Geometry check sheet. Reference: the model listing, model coordinates, mm. Face numbers are marked on the shaded views. A direction names the side the tool comes from. Give positions to 0.01 mm unless a question says otherwise; leave off trailing zeros. Order: outer loops, then holes, each group sorted by start corner. A loop starts at its lowest first (then second) coordinate and runs counter-clockwise, first axis right, second up.
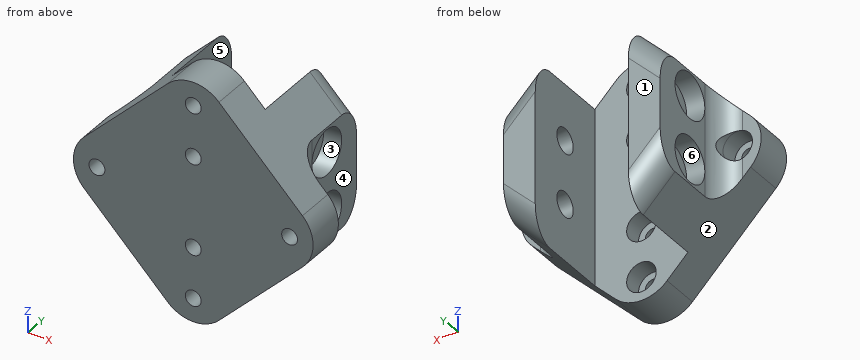
from build123d import *

# Parameters (mm, degrees)
SKETCH_1_R          = 1.75
EXTRUDE_1_DEPTH     = 8.5
EXTRUDE_2_DEPTH     = 20
SKETCH_3_R          = 2.75
CUT_EXTRUDE_1_DEPTH = 59.415752368
SKETCH_4_R          = 5
CUT_EXTRUDE_2_DEPTH = 4
SKETCH_5_R          = 3.25
CUT_EXTRUDE_3_DEPTH = 4
FILLET_2_R          = 5


with BuildPart() as part:
    # Эскиз1 → Бобышка-Вытянуть1 (new body)
    with BuildSketch(Plane(origin=(0, 0, 0), x_dir=(1, 0, 0), z_dir=(0, 1, 0))):
        with BuildLine():
            Line((5.656854249, -24.04163056), (24.04163056, -5.656854249))
            ThreePointArc((24.04163056, -5.656854249), (26.384776311, 0), (24.04163056, 5.656854249))
            Line((24.04163056, 5.656854249), (5.656854249, 24.04163056))
            ThreePointArc((5.656854249, 24.04163056), (0, 26.384776311), (-5.656854249, 24.04163056))
            Line((-5.656854249, 24.04163056), (-24.04163056, 5.656854249))
            ThreePointArc((-24.04163056, 5.656854249), (-26.384776311, 0), (-24.04163056, -5.656854249))
            Line((-24.04163056, -5.656854249), (-5.656854249, -24.04163056))
            ThreePointArc((-5.656854249, -24.04163056), (0, -26.384776311), (5.656854249, -24.04163056))
        make_face()
        with Locations(Location((21.213203436, 0, 0), (0, 0, 270))):
            Circle(SKETCH_1_R, mode=Mode.SUBTRACT)
        with Locations(Location((0, -10, 0), (0, 0, 270))):
            Circle(SKETCH_1_R, mode=Mode.SUBTRACT)
        with Locations(Location((0, -21.213203436, 0), (0, 0, 270))):
            Circle(SKETCH_1_R, mode=Mode.SUBTRACT)
        with Locations(Location((-21.213203436, 0, 0), (0, 0, 270))):
            Circle(SKETCH_1_R, mode=Mode.SUBTRACT)
        with Locations(Location((0, 10, 0), (0, 0, 270))):
            Circle(SKETCH_1_R, mode=Mode.SUBTRACT)
        with Locations(Location((0, 21.213203436, 0), (0, 0, 270))):
            Circle(SKETCH_1_R, mode=Mode.SUBTRACT)
    extrude(amount=EXTRUDE_1_DEPTH)

    # Эскиз2 → Бобышка-Вытянуть2 (add)
    with BuildSketch(Plane(origin=(0, 8.5, 0), x_dir=(1, 0, 0), z_dir=(0, 1, 0))):
        Polygon((-10.25, 19.44848481), (-10.25, -19.44848481), (-17.25, -12.44848481), (-17.25, 12.44848481), align=None)
        Polygon((17.25, 12.44848481), (10.25, 19.44848481), (10.25, -19.44848481), (17.25, -12.44848481), align=None)
    extrude(amount=EXTRUDE_2_DEPTH)

    # Эскиз3 → Вырез-Вытянуть1 (cut, through all)
    with BuildSketch(Plane(origin=(17.25, 0, 0), x_dir=(0, 0, -1), z_dir=(1, 0, 0))):
        with Locations((-7, 18.5)):
            Circle(SKETCH_3_R)
        with Locations((7, 18.5)):
            Circle(SKETCH_3_R)
    extrude(amount=-CUT_EXTRUDE_1_DEPTH, mode=Mode.SUBTRACT)

    # Эскиз4 → Вырез-Вытянуть2 (cut)
    with BuildSketch(Plane(origin=(17.25, 0, 0), x_dir=(0, 0, -1), z_dir=(1, 0, 0))):
        with Locations((-7, 18.5)):
            Circle(SKETCH_4_R)
        with Locations((7, 18.5)):
            Circle(SKETCH_4_R)
    cut_extrude_2 = extrude(amount=-CUT_EXTRUDE_2_DEPTH, mode=Mode.SUBTRACT)

    # Зеркальное отражение1: Вырез-Вытянуть2 across plane
    add(cut_extrude_2.mirror(Plane(origin=(0, 0, 0), x_dir=(0, 0, 1), z_dir=(1, 0, 0))), mode=Mode.SUBTRACT)

    # Эскиз5 → Вырез-Вытянуть3 (cut)
    with BuildSketch(Plane(origin=(0, 8.5, 0), x_dir=(1, 0, 0), z_dir=(0, 1, 0))):
        with Locations(Location((0, 21.213203436, 0), (0, 0, 270))):
            Circle(SKETCH_5_R)
        with Locations(Location((0, 10, 0), (0, 0, 270))):
            Circle(SKETCH_5_R)
        with Locations(Location((0, -10, 0), (0, 0, 270))):
            Circle(SKETCH_5_R)
        with Locations(Location((0, -21.213203436, 0), (0, 0, 270))):
            Circle(SKETCH_5_R)
        with Locations(Location((21.213203436, 0, 0), (0, 0, 270))):
            Circle(SKETCH_5_R)
        with Locations(Location((-21.213203436, 0, 0), (0, 0, 270))):
            Circle(SKETCH_5_R)
    extrude(amount=-CUT_EXTRUDE_3_DEPTH, mode=Mode.SUBTRACT)

    # Скругление2
    # the kernel refuses this fillet: 5 mm, written as the material it adds along each edge
    with BuildSketch(Plane(origin=(-17.25, 8.5, 24.94848481), x_dir=(-1, 0, 0), z_dir=(0, 0, -1))) as fillet_2_piece_1_section:
        with BuildLine():
            CenterArc((FILLET_2_R, FILLET_2_R), FILLET_2_R, 180, 90)
            Line((0, FILLET_2_R), (0, 0))
            Line((0, 0), (FILLET_2_R, 0))
        make_face()
    fillet_2_piece_1 = extrude(amount=49.89696962, mode=Mode.PRIVATE)
    fillet_2_piece_1 = split(fillet_2_piece_1, bisect_by=Plane(origin=(-29.470144139, 8.621513924, 0.22834067), z_dir=(0.7071067811865474, 0, -0.7071067811865477)), keep=Keep.TOP, mode=Mode.PRIVATE)
    fillet_2_piece_1 = split(fillet_2_piece_1, bisect_by=Plane(origin=(-21.171154266, 8.621513924, -8.527330544), z_dir=(0.7071067811865477, 0, 0.7071067811865474)), keep=Keep.TOP, mode=Mode.PRIVATE)
    fillet_2_piece_1 = fillet_2_piece_1 - Plane(origin=(-21.213203436, 8.621513924, 0), x_dir=(0, 0, 1), z_dir=(0, 1, 0)) * Cylinder(3.25, 120, mode=Mode.PRIVATE)
    add(fillet_2_piece_1)
    with BuildSketch(Plane(origin=(17.25, 8.5, 24.94848481), x_dir=(0, 1, 0), z_dir=(0, 0, -1))) as fillet_2_piece_2_section:
        with BuildLine():
            CenterArc((FILLET_2_R, FILLET_2_R), FILLET_2_R, 180, 90)
            Line((0, FILLET_2_R), (0, 0))
            Line((0, 0), (FILLET_2_R, 0))
        make_face()
    fillet_2_piece_2 = extrude(amount=49.89696962, mode=Mode.PRIVATE)
    fillet_2_piece_2 = split(fillet_2_piece_2, bisect_by=Plane(origin=(27.68449432, 12.192813605, 2.013990489), z_dir=(-0.7071067811865477, 0, -0.7071067811865474)), keep=Keep.TOP, mode=Mode.PRIVATE)
    fillet_2_piece_2 = split(fillet_2_piece_2, bisect_by=Plane(origin=(19.385504447, 12.192813605, -10.312980363), z_dir=(-0.7071067811865472, 0, 0.7071067811865478)), keep=Keep.TOP, mode=Mode.PRIVATE)
    fillet_2_piece_2 = fillet_2_piece_2 - Plane(origin=(21.213203436, 12.192813605, 0), x_dir=(0, 0, 1), z_dir=(0, 1, 0)) * Cylinder(3.25, 120, mode=Mode.PRIVATE)
    add(fillet_2_piece_2)
    # the kernel refuses this fillet: 5 mm, written as the material it takes off along each edge
    with BuildSketch(Plane(origin=(-26.088834765, 28.5, -3.609650045), x_dir=(0, -1, 0), z_dir=(0.7071067811865472, 0, -0.7071067811865478)), Plane(origin=(1.411165235, 28.5, 28.287319575), x_dir=(-0.7071067811865474, 0, -0.7071067811865477), z_dir=(0.7071067811865477, 0, -0.7071067811865474))) as fillet_2_2_piece_1:
        with BuildLine():
            CenterArc((FILLET_2_R, -FILLET_2_R), FILLET_2_R, 90, 90)
            Line((0, -FILLET_2_R), (0, 0))
            Line((0, 0), (FILLET_2_R, 0))
        make_face()
    extrude(amount=34.899494937, mode=Mode.SUBTRACT)
    with BuildSketch(Plane(origin=(-1.411165235, 28.5, 28.287319575), x_dir=(0.7071067811865474, 0, -0.7071067811865477), z_dir=(-0.7071067811865477, 0, -0.7071067811865474)), Plane(origin=(26.088834765, 28.5, -3.609650045), x_dir=(0, -1, 0), z_dir=(-0.7071067811865472, 0, -0.7071067811865478))) as fillet_2_2_piece_2:
        with BuildLine():
            CenterArc((FILLET_2_R, FILLET_2_R), FILLET_2_R, 180, 90)
            Line((0, FILLET_2_R), (0, 0))
            Line((0, 0), (FILLET_2_R, 0))
        make_face()
    extrude(amount=34.899494937, mode=Mode.SUBTRACT)


solid = part.part
Item 1: Sectioned sample at C-C (x = 0). Give the number of separate pieces and of enclosed holes in the cut face, and give its area (3 significant figures).
Reported:
separate pieces: 5
enclosed holes: 0
area: 282 mm2
Item 2: Sectioned sample at B-B (y = 26.25). Enter the section's corners in (x, z).
Reported:
outline: (-17.25, -11.28) - (-10.25, -18.28) - (-10.25, 18.28) - (-17.25, 11.28) - close; (10.25, -18.28) - (17.25, -11.28) - (17.25, 11.28) - (10.25, 18.28) - close
Item 3: Draft check along Y on the marked faces 1, 2 and 3. Enter one of: released by +Y, released by -Y, zero draft, split by the parting line, or undercut.
Reported:
face 1: released by +Y
face 2: zero draft
face 3: undercut
Item 4: Sectioned sample at A-A (z = 0). Enter the section's corners in (x, y), and give its area (3 significant figures).
Reported:
outline: (-26.38, 0) - (-22.96, 0) - (-22.96, 4.5) - (-24.46, 4.5) - (-24.46, 8.5) - (-26.38, 8.5) - close; (-19.46, 0) - (19.46, 0) - (19.46, 4.5) - (17.96, 4.5) - (17.96, 10.93) arc R5 cw to (17.25, 13.5) - (17.25, 28.5) - (10.25, 28.5) - (10.25, 8.5) - (-10.25, 8.5) - (-10.25, 28.5) - (-17.25, 28.5) - (-17.25, 13.5) arc R5 cw to (-17.96, 10.93) - (-17.96, 4.5) - (-19.46, 4.5) - close; (22.96, 0) - (26.38, 0) - (26.38, 8.5) - (24.46, 8.5) - (24.46, 4.5) - (22.96, 4.5) - close
area: 650 mm2
Item 5: Scan lines: L1, parallel to Z at x = 0, y = 3.55; L2, parallel to Y at x = 12.2, z = 7; L3, parallel to Y at x = 14.35, z = -7. Record each from-to range of solid material in increasing order.
Reported:
L1: z = -26.38 to -22.96, -19.46 to -11.75, -8.25 to 8.25, 11.75 to 19.46, 22.96 to 26.38
L2: y = 0 to 15.75, 21.25 to 28.5
L3: y = 0 to 13.5, 23.5 to 28.5
Item 6: Set-up check for the marked faces 4, 5 and 6: record each of +Z, -Z, +X, -X, +Y, -Y from which the full face is reachable in a straight line by a thin tool's end or side.
Reported:
face 4: +Z, -Z, +X, +Y
face 5: +Z, -Z, +Y
face 6: -X
Item 7: Gauge pin test, flat ends, axial feed: pin 1 (7 mm diameter, centred on x = -0.5, z = 9.5, fed in from +Y); pin 2 (5 mm diameter, centred on y = 13, z = 0, fed in from +X); pin 3 (8 mm diameter, centred on x = -12.5, y = 7.5, fed in from +Z). Record the tip position at first contact, or that the pin passes through.
Reported:
pin 1: stops at y = 8.5
pin 2: stops at x = 18.11
pin 3: stops at z = 21.2
